The listing builds one solid part. Answer for the finished solid, in the listing's coordinates (mm). A direction names the side the tool comes from. Coordinates: 2 decimals unless noted, no trailing zeros. Order: outer loops, then holes, each group sorted by start corner. A loop starts at its lowest first (then second) coordinate and runs counter-clockwise, first axis right, second up.
Autodesk Inventor part; units mm, degrees
ref_plane "YZ Plane" through (0, 0, 0) normal (1, 0, 0) x (0, 1, 0)
ref_plane "XZ Plane" through (0, 0, 0) normal (0, 1, 0) x (-1, 0, 0)
ref_plane "XY Plane" through (0, 0, 0) normal (0, 0, 1) x (1, 0, 0)
sketch "Sketch1" plane through (0, 0, 0) normal (0, 1, 0) x (-1, 0, 0)
  line L0 (-11, 14.2) -> (-11, -14.2)
  line L1 (-10, -15.2) -> (10, -15.2)
  line L2 (11, -14.2) -> (11, 14.2)
  line L3 (10, 15.2) -> (-10, 15.2)
  line L4 (-11, 15.2) -> (11, -15.2) construction
  line L5 (-11, -15.2) -> (11, 15.2) construction
  line L6 (-10, 13.2) -> (-10, -13.2)
  line L7 (-9, -14.2) -> (9, -14.2)
  line L8 (10, -13.2) -> (10, 13.2)
  line L9 (9, 14.2) -> (-9, 14.2)
  line L10 (-10, 14.2) -> (10, -14.2) construction
  line L11 (-10, -14.2) -> (10, 14.2) construction
  arc A0 (11, 14.2) -> (10, 15.2) centre (10, 14.2) ccw
  arc A1 (10, 13.2) -> (9, 14.2) centre (9, 13.2) ccw
  arc A2 (9, -14.2) -> (10, -13.2) centre (9, -13.2) ccw
  arc A3 (10, -15.2) -> (11, -14.2) centre (10, -14.2) ccw
  arc A4 (-10, -13.2) -> (-9, -14.2) centre (-9, -13.2) ccw
  arc A5 (-11, -14.2) -> (-10, -15.2) centre (-10, -14.2) ccw
  arc A6 (-10, 15.2) -> (-11, 14.2) centre (-10, 14.2) ccw
  arc A7 (-9, 14.2) -> (-10, 13.2) centre (-9, 13.2) ccw
  point P0 (0, 0)
  dimension "d0" = 30.4
  dimension "d1" = 22
  dimension "d2" = 28.4
  dimension "d3" = 20
  dimension "d4" = 1
  dimension "d5" = 1
extrude "Extrusion1" add sketch "Sketch1" along normal blind 18
sketch "Sketch3" plane through (-9, 0, -14.2) normal (0, 0, 1) x (1, 0, 0)
  line L0 (9, 0) -> (9, 9)
  circle A0 centre (9, 9) radius 9
  dimension "d12" = 9
  dimension "d13" = 18
extrude "Extrusion3" add sketch "Sketch3" along normal up to surface (28.4 mm away)
sketch "Sketch4" plane through (-10, 0, 15.2) normal (0, 0, 1) x (1, 0, 0)
  circle A0 centre (10, 9) radius 4
  point P0 (10, 0)
  dimension "d16" = 8
extrude "Extrusion4" add sketch "Sketch4" along normal blind 10
sketch "Sketch5" plane through (0, 9, 25.2) normal (0, 0, 1) x (1, 0, 0)
  circle A0 centre (0, 0) radius 5
  point P0 (0, -9)
  dimension "d19" = 10
extrude "Extrusion5" add sketch "Sketch5" along normal blind 1
sketch "Sketch7" plane through (10, 0, -15.2) normal (0, 0, -1) x (-1, 0, 0)
  line L0 (10, 9) -> (10, 0)
  circle A0 centre (10, 9) radius 1.75
  dimension "d22" = 3.5
extrude "Extrusion6" add sketch "Sketch7" along normal blind 9
sketch "Sketch8" plane through (11, 0, 14.2) normal (1, 0, 0) x (0, 0, -1)
  line L0 (-1, 0) -> (-1, 18)
  line L1 (-1, 9) -> (5.5, 9)
  line L2 (5.5, 9) -> (5.5, 14)
  line L3 (5.5, 14) -> (5.5, 4)
  line L4 (5.5, 4) -> (13.5, 4)
  line L5 (13.5, 4) -> (13.5, 14)
  circle A0 centre (5.5, 14) radius 1.5
  circle A1 centre (13.5, 14) radius 1.5
  circle A2 centre (13.5, 4) radius 1.5
  circle A3 centre (5.5, 4) radius 1.5
  point P0 (14.2, 0)
  dimension "d25" = 6.5
  dimension "d26" = 5
  dimension "d27" = 10
  dimension "d28" = 8
  dimension "d29" = 3
  dimension "d30" = 3
  dimension "d31" = 3
  dimension "d32" = 3
extrude "Extrusion7" cut sketch "Sketch8" against normal blind 2
properties part number "Solenoid"
1) A cutting plane is placed at D-D, the plane x = 6.5. Write down the section's boundary in (y, z), plus the area to 3 significant figures.
2) A cutting plane is placed at C-C, the plane y = 4.5. Count the separate pieces of the cut face and the enclosed holes in it, plus the area to 3 significant figures.
3) A cutting plane is placed at A-A, the plane z = 8.7. Write down the section's boundary in (x, y), plus the area to 3 significant figures.
4) For faces 1 (the flat face through (-7, 16, -14.2)), 2 (the flat face through (-7, 2, 14.2)), 3 (the cylindrical face through (10.51, 4.45, 7.27)), 4 (the cylindrical face through (-7.14, 14.48, -0.2)), determine the directions among +Z, -Z, +X, -X, +Y, -Y from which every point of the face is accessible in a straight line to the end or side of a thin tool.
5) A cutting plane is placed at B-B, the plane y = 15. Write down the section's boundary in (x, z).
6) Straight lines are drawn through the part: probe 1 along Y at (x, z) = (10.35, 8.7); probe 2 along X at (y, z) = (6, 6); probe 3 along X at (y, z) = (5, 10). For each, find the intervals that lie inside material, in ascending order.
7) Each of these flat-tipped pins is pushed along its axis until it touches: P1, Ø5, axis at x = 1.5, y = 16, coming from the -Z side; P2, Ø2.5, axis at x = 5.5, y = 5, coming from the +Z side; P3, Ø2, axis at y = 5, z = 18.5, coming from the +X side. Where does it stop, or does it pass through?
8) The mould has two halves that part along Z. Classify faces 5 (the cylindrical face through (0.228, 7.265, -19.637)), 6 (the flat face through (0, 9, -24.2)), 7 (the flat face through (10, 9, 0)): released by +Z, released by -Z, zero draft, split by the parting line, or undercut.
Working result:
1. outline: (0, -15.2) - (18, -15.2) - (18, -14.2) - (15.22, -14.2) - (15.22, 14.2) - (18, 14.2) - (18, 15.2) - (0, 15.2) - (0, 14.2) - (2.78, 14.2) - (2.78, -14.2) - (0, -14.2) - close
1. area: 390 mm2
2. separate pieces: 3
2. enclosed holes: 1
2. area: 542 mm2
3. outline: (-11, 0) - (-10, 0) - (-10, 18) - (-11, 18) - close; circle Ø18 at (0, 9); (10, 0) - (11, 0) - (11, 2.5) - (10, 2.5) - close; (10, 5.5) - (11, 5.5) - (11, 12.5) - (10, 12.5) - close; (10, 15.5) - (11, 15.5) - (11, 18) - (10, 18) - close
3. area: 284 mm2
4. face 1: +Y
4. face 2: -Y
4. face 3: +X
4. face 4: none
5. outline: (-11, -14.2) arc R1 ccw to (-10, -15.2) - (10, -15.2) arc R1 ccw to (11, -14.2) - (11, -0.42) - (10, -0.42) - (10, -13.2) arc R1 cw to (9, -14.2) - (6.71, -14.2) - (6.71, 14.2) - (9, 14.2) arc R1 cw to (10, 13.2) - (10, 9.82) - (11, 9.82) - (11, 14.2) arc R1 ccw to (10, 15.2) - (-10, 15.2) arc R1 ccw to (-11, 14.2) - close; (10, 1.82) - (11, 1.82) - (11, 7.58) - (10, 7.58) - close; hole (-10, -13.2) arc R1 ccw to (-9, -14.2) - (-6.71, -14.2) - (-6.71, 14.2) - (-9, 14.2) arc R1 ccw to (-10, 13.2) - close
6. probe 1: y = 0 to 2.5, 5.5 to 12.5, 15.5 to 18
6. probe 2: x = -11 to -10, -8.49 to 8.49, 10 to 11
6. probe 3: x = -11 to -10, -8.06 to 8.06, 10 to 11
7. P1: stops at z = -15.2
7. P2: stops at z = 15.2
7. P3: stops at x = 2.65
8. face 5: zero draft
8. face 6: released by -Z
8. face 7: undercut
